Job drawing, mm, ordinate dimensions from the low corner. One solid piece. A direction names the side the tool comes from. Coordinates: 2 decimals unless noted, no trailing zeros. Order: outer loops, then holes, each group sorted by start corner. A loop starts at its lowest first (then second) coordinate and runs counter-clockwise, first axis right, second up. Notation, with made-up numbers: M -21.5,11 L 3.5,11 A22 ccw 3.5,47 Z; hole C 70.25,43.25 d8. An arc over 180 degrees is marked long. Write item = value, one per line.
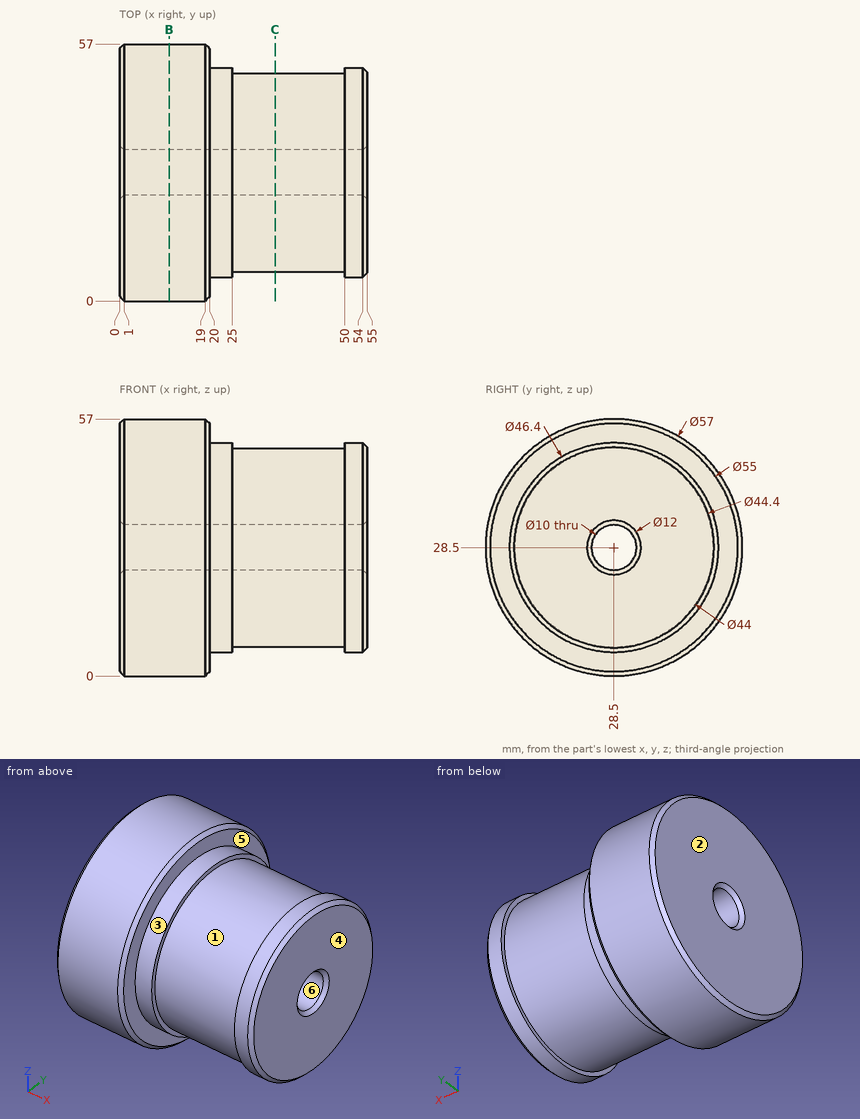
(1) Wall check: line 1 (Y direction, x = 29, z = 28.5); line 2 (Y direction, x = 16.5, z = 28.5); line 3 (X direction, y = 9, z = 14.5). Give the ranges that are in metal, low to high. Write a range as from..to.
Evaluation:
line_1 = 6.5..23.5, 33.5..50.5
line_2 = 0..23.5, 33.5..57
line_3 = 0..20
(2) Pin check, flat tips, straight feed: pin 1 Ø2 at (x, z) = (26.5, 24) entering from +Y; pin 2 Ø5 at (y, z) = (45, 10) entering from +X; pin 3 Ø8 at (x, z) = (45, 36) entering from -Y; pin 4 Ø10 at (y, z) = (19.5, 27) entering from -X. Stop position of each tip, or through.
Evaluation:
pin_1 = 50.22
pin_2 = 54.91
pin_3 = 6.78
pin_4 = 0
(3) Tool access for the marked faces 5 and 6: list every direction of +Z, -Z, +X, -X, +Y, -Y with a clear straight run to the whole face (end or side of a thin tool).
Evaluation:
face_5 = +X
face_6 = +X, -X
(4) Slice it at C-C, the plane x = 34.5. Write the cut outline in (y, z).
Evaluation:
outline = C 28.5,28.5 d44; hole C 28.5,28.5 d10
(5) Slice it at B-B, the plane x = 11. Write the cut outline in (y, z).
Evaluation:
outline = C 28.5,28.5 d57; hole C 28.5,28.5 d10
(6) Pull direction X, two halves, no side cores. Call the marked faces 1, 2, 3 and 4: +X half, -X half, draft (parallel to the pull), parting line (faces both ways), or undercut.
Evaluation:
face_1 = undercut
face_2 = -X half
face_3 = draft
face_4 = +X half
